```python
from build123d import *

# Parameters (mm, degrees)
SKETCH1_W            = 6.266
SKETCH1_H            = 19.6
SKETCH1_R            = 1.675
SKETCH1_W_2          = 52.832
SKETCH1_H_2          = 5
BOSS_EXTRUDE2_DEPTH  = 3.175
SKETCH3_W            = 30
SKETCH3_H            = 29.6
BOSS_EXTRUDE3_DEPTH  = 3.175
SKETCH4_R            = 4.75
CUT_EXTRUDE1_DEPTH   = 10
BOSS_EXTRUDE14_DEPTH = 3.175
CUT_EXTRUDE8_DEPTH   = 10
SKETCH24_R           = 1.475
CUT_EXTRUDE9_DEPTH   = 10
SKETCH25_R           = 3.675
SKETCH25_R_2         = 1.675
BOSS_EXTRUDE15_DEPTH = 3.175
SKETCH26_R           = 1.475
CUT_EXTRUDE12_DEPTH  = 3.175
CUT_EXTRUDE13_DEPTH  = 10
SKETCH28_R           = 3.675
SKETCH28_R_2         = 1.675
BOSS_EXTRUDE16_DEPTH = 3.175
SKETCH29_R           = 1.475
BOSS_EXTRUDE17_DEPTH = 3.175
SKETCH30_W           = 52.236337303
SKETCH30_H           = 21.491937942
BOSS_EXTRUDE18_DEPTH = 3.175
CUT_EXTRUDE14_DEPTH  = 10
SKETCH32_R           = 1.475
BOSS_EXTRUDE19_DEPTH = 4
SKETCH33_R           = 2.220955703
SKETCH33_R_2         = 1.475
SKETCH33_R_3         = 2.214708119
BOSS_EXTRUDE20_DEPTH = 3.175
SKETCH34_R           = 1.475
BOSS_EXTRUDE21_DEPTH = 4


with BuildPart() as part:
    # Sketch1 → Boss-Extrude2 (new body)
    # profile 1 of 4: a face of its own
    with BuildSketch(Plane.XY):
        with Locations((-23.283, 0)):
            Rectangle(SKETCH1_W, SKETCH1_H)
        with Locations((-23.95, -4.974)):
            Circle(SKETCH1_R, mode=Mode.SUBTRACT)
        with Locations((-23.95, 4.974)):
            Circle(SKETCH1_R, mode=Mode.SUBTRACT)
    # profile 2 of 4: a face of its own
    with BuildSketch(Plane.XY):
        with Locations((0, -12.3)):
            Rectangle(SKETCH1_W_2, SKETCH1_H_2)
    # profile 3 of 4: a face of its own
    with BuildSketch(Plane.XY):
        with Locations((0, 12.3)):
            Rectangle(SKETCH1_W_2, SKETCH1_H_2)
    # profile 4 of 4: a face of its own
    with BuildSketch(Plane.XY):
        with Locations((23.283, 0)):
            Rectangle(SKETCH1_W, SKETCH1_H)
        with Locations((23.95, -4.974)):
            Circle(SKETCH1_R, mode=Mode.SUBTRACT)
        with Locations((23.95, 4.974)):
            Circle(SKETCH1_R, mode=Mode.SUBTRACT)
    extrude(amount=BOSS_EXTRUDE2_DEPTH)

    # Sketch3 → Boss-Extrude3 (add)
    with BuildSketch(Plane.XY.offset(3.175)):
        with Locations((41.416, 0)):
            Rectangle(SKETCH3_W, SKETCH3_H)
    extrude(amount=-BOSS_EXTRUDE3_DEPTH)

    # Sketch4 → Cut-Extrude1 (cut)
    with BuildSketch(Plane(origin=(0, 0, 0), x_dir=(-1, 0, 0), z_dir=(0, 0, -1))):
        with Locations((-40.576, 7.77)):
            Circle(SKETCH4_R)
    extrude(amount=-CUT_EXTRUDE1_DEPTH, mode=Mode.SUBTRACT)

    # Sketch22 → Boss-Extrude14 (add)
    with BuildSketch(Plane(origin=(0, 0, 0), x_dir=(-1, 0, 0), z_dir=(0, 0, -1))):
        with BuildLine():
            ThreePointArc((-34.680262133, 14.8), (-40.576, 16.945), (-46.471737867, 14.8))
            Line((-46.471737867, 14.8), (-34.680262133, 14.8))
        make_face()
    extrude(amount=-BOSS_EXTRUDE14_DEPTH)

    # Sketch23 → Cut-Extrude8 (cut)
    with BuildSketch(Plane(origin=(0, 0, 0), x_dir=(-1, 0, 0), z_dir=(0, 0, -1))):
        with BuildLine():
            Line((-49.751, -14.8), (-49.751, 7.77))
            ThreePointArc((-49.751, 7.77), (-48.890866804, 11.648609936), (-46.471737867, 14.8))
            Line((-46.471737867, 14.8), (-56.416, 14.8))
            Line((-56.416, 14.8), (-56.416, -14.8))
            Line((-56.416, -14.8), (-49.751, -14.8))
        make_face()
    extrude(amount=-CUT_EXTRUDE8_DEPTH, mode=Mode.SUBTRACT)

    # Sketch24 → Cut-Extrude9 (cut)
    with BuildSketch(Plane(origin=(0, 0, 0), x_dir=(-1, 0, 0), z_dir=(0, 0, -1))):
        with Locations((23.736, 13.59)):
            Circle(SKETCH24_R)
    extrude(amount=-CUT_EXTRUDE9_DEPTH, mode=Mode.SUBTRACT)

    # Sketch25 → Boss-Extrude15 (add)
    # profile 1 of 3: a face of its own
    with BuildSketch(Plane(origin=(0, 0, 0), x_dir=(-1, 0, 0), z_dir=(0, 0, -1))):
        with Locations((23.95, -4.974)):
            Circle(SKETCH25_R)
        with Locations(Location((23.95, -4.974, 0), (0, 0, 180))):
            Circle(SKETCH25_R_2, mode=Mode.SUBTRACT)
    # profile 2 of 3: a face of its own
    with BuildSketch(Plane(origin=(0, 0, 0), x_dir=(-1, 0, 0), z_dir=(0, 0, -1))):
        with Locations((23.95, 4.974)):
            Circle(SKETCH25_R)
        with Locations(Location((23.95, 4.974, 0), (0, 0, 180))):
            Circle(SKETCH25_R_2, mode=Mode.SUBTRACT)
    # profile 3 of 3: a face of its own
    with BuildSketch(Plane(origin=(0, 0, 0), x_dir=(-1, 0, 0), z_dir=(0, 0, -1))):
        with Locations((23.736, 13.59)):
            Circle(SKETCH25_R)
        with Locations((23.736, 13.59)):
            Circle(SKETCH25_R_2, mode=Mode.SUBTRACT)
    extrude(amount=-BOSS_EXTRUDE15_DEPTH)

    # Sketch26 → Cut-Extrude12 (cut)
    with BuildSketch(Plane(origin=(0, 0, 0), x_dir=(-1, 0, 0), z_dir=(0, 0, -1))):
        with Locations((-46.076, -11.125)):
            Circle(SKETCH26_R)
    extrude(amount=-CUT_EXTRUDE12_DEPTH, mode=Mode.SUBTRACT)

    # Sketch27 → Cut-Extrude13 (cut)
    with BuildSketch(Plane(origin=(0, 0, 0), x_dir=(-1, 0, 0), z_dir=(0, 0, -1))):
        with BuildLine():
            ThreePointArc((-22.190754209, 13.59), (-22.358119678, 14.272434563), (-22.822234796, 14.8))
            Line((-22.822234796, 14.8), (-24.509273622, 14.8))
            ThreePointArc((-24.509273622, 14.8), (-24.348188772, 12.282365469), (-22.190754209, 13.59))
        make_face()
        with BuildLine():
            Line((-24.509273622, 14.8), (-22.822234796, 14.8))
            ThreePointArc((-22.822234796, 14.8), (-23.665754209, 15.065), (-24.509273622, 14.8))
        make_face()
    extrude(amount=-CUT_EXTRUDE13_DEPTH, mode=Mode.SUBTRACT)

    # Sketch28 → Boss-Extrude16 (add)
    with BuildSketch(Plane(origin=(0, 0, 0), x_dir=(-1, 0, 0), z_dir=(0, 0, -1))):
        with Locations((-23.665754209, 13.59)):
            Circle(SKETCH28_R)
        with Locations((-23.665754209, 13.59)):
            Circle(SKETCH28_R_2, mode=Mode.SUBTRACT)
    extrude(amount=-BOSS_EXTRUDE16_DEPTH)

    # Sketch29 → Boss-Extrude17 (add)
    with BuildSketch(Plane(origin=(0, 0, 0), x_dir=(-1, 0, 0), z_dir=(0, 0, -1))):
        with BuildLine():
            ThreePointArc((35.566, -11.125), (32.517318638, -5.113632727), (26.416, -2.249212118))
            Line((26.416, -2.249212118), (26.416, -14.8))
            Line((26.416, -14.8), (32.091, -14.6))
            ThreePointArc((32.091, -14.6), (34.548196065, -13.582196065), (35.566, -11.125))
        make_face()
        with Locations((32.091, -11.125)):
            Circle(SKETCH29_R, mode=Mode.SUBTRACT)
    extrude(amount=-BOSS_EXTRUDE17_DEPTH)

    # Sketch30 → Boss-Extrude18 (add)
    with BuildSketch(Plane(origin=(0, 0, 0), x_dir=(-1, 0, 0), z_dir=(0, 0, -1))):
        with Locations((-0.180648482, 0.066835569)):
            Rectangle(SKETCH30_W, SKETCH30_H)
    extrude(amount=-BOSS_EXTRUDE18_DEPTH)

    # Sketch31 → Cut-Extrude14 (cut)
    with BuildSketch(Plane(origin=(0, 0, 0), x_dir=(-1, 0, 0), z_dir=(0, 0, -1))):
        Polygon((26.416, 9.86570219), (26.416, 0.686094798), (31.474426215, 3.163131713), align=None)
    extrude(amount=-CUT_EXTRUDE14_DEPTH, mode=Mode.SUBTRACT)

    # Sketch32 → Boss-Extrude19 (add)
    with BuildSketch(Plane(origin=(0, -14.8, 0), x_dir=(-1, 0, 0), z_dir=(0, -1, 0))):
        with BuildLine():
            ThreePointArc((-22.83, -3.175), (-16.387108849, -7.772233652), (-8.83, -10.125))
            ThreePointArc((-8.83, -10.125), (-1.272891151, -7.772233652), (5.17, -3.175))
            Line((5.17, -3.175), (-22.83, -3.175))
        make_face()
        with Locations(Location((-8.83, -6.65, 0), (0, 0, 180))):
            Circle(SKETCH32_R, mode=Mode.SUBTRACT)
    extrude(amount=-BOSS_EXTRUDE19_DEPTH)

    # Sketch33 → Boss-Extrude20 (add)
    # profile 1 of 2: a face of its own
    with BuildSketch(Plane(origin=(0, 0, 0), x_dir=(-1, 0, 0), z_dir=(0, 0, -1))):
        with Locations((-23.665754209, 13.59)):
            Circle(SKETCH33_R)
        with Locations((-23.665754209, 13.59)):
            Circle(SKETCH33_R_2, mode=Mode.SUBTRACT)
    # profile 2 of 2: a face of its own
    with BuildSketch(Plane(origin=(0, 0, 0), x_dir=(-1, 0, 0), z_dir=(0, 0, -1))):
        with Locations((23.736, 13.59)):
            Circle(SKETCH33_R_3)
        with Locations((23.736, 13.59)):
            Circle(SKETCH33_R_2, mode=Mode.SUBTRACT)
    extrude(amount=-BOSS_EXTRUDE20_DEPTH)

    # Sketch34 → Boss-Extrude21 (add)
    with BuildSketch(Plane(origin=(0, -14.8, 0), x_dir=(-1, 0, 0), z_dir=(0, -1, 0))):
        with BuildLine():
            Line((5.17, -3.175), (-22.83, -3.175))
            ThreePointArc((-22.83, -3.175), (-8.83, -10.125), (5.17, -3.175))
        make_face()
        with Locations(Location((-8.83, -6.65, 0), (0, 0, 180))):
            Circle(SKETCH34_R, mode=Mode.SUBTRACT)
    extrude(amount=-BOSS_EXTRUDE21_DEPTH)


solid = part.part
```
For this review, take the finished solid that the model builds, in its own axes (mm). A direction names the side the tool comes from. Round coordinates to 2 decimals unless told otherwise and drop trailing zeros. Write each loop counter-clockwise with the first axis right and the second up, starting at its lowest first coordinate (ties: lowest second). Pieces come first, ordered by that corner, then holes. Notation, with made-up numbers: (56, -16.5) - (110, -16.5) arc R9 ccw to (110, -12.5) - close; hole circle Ø9 at (42.25, -17). An arc over 180 degrees is marked (long way). Answer as a JSON object with one key per item and string values.
1. We need section B-B on y = 5.5. Give the boundary of the cut face in (x, z) (3 decimals), then the cut area to 3 significant figures.
Response values:
{"outline": "(-26.416, 0) - (36.404, 0) - (36.404, 3.175) - (-26.416, 3.175) - close; (44.748, 0) - (49.751, 0) - (49.751, 3.175) - (44.748, 3.175) - close", "area": "215 mm2"}
2. Draft analysis for pull direction Z (two halves, no side actions). For faces 1 (the face through (-25.717, 16.685, 1.565)), 2 (the face through (8, 1, 3.175)), 3 (the face through (10.2, -12.8, 6.1)), state which applies: +Z half, -Z half, draft (parallel to the pull), parting line (faces both ways), or undercut.
Response values:
{"face 1": "draft", "face 2": "+Z half", "face 3": "undercut"}
3. We need section A-A on x = 8.83. Give the boundary of the cut face in (y, z) (3 decimals), then the cut area to 3 significant figures.
Response values:
{"outline": "(-14.8, 0) - (14.8, 0) - (14.8, 3.175) - (-10.8, 3.175) - (-10.8, 5.175) - (-14.8, 5.175) - close; (-14.8, 8.125) - (-10.8, 8.125) - (-10.8, 10.125) - (-14.8, 10.125) - close", "area": "110 mm2"}
4. Tool access review of faces 4 (the face through (0, 14.8, 2)), 5 (the face through (-26.416, 4, 2)), 6 (the face through (11, -14.8, 3)): name each direction out of +Z, -Z, +X, -X, +Y, -Y from which nothing blocks a thin tool from reaching the whole face with its end or side.
Response values:
{"face 4": "+Z, -Z, +Y", "face 5": "+Z, -Z, -X", "face 6": "+Z, -Z, +X, -X, -Y"}
5. To check wall thickness, follow line 1 along X through (y, z) = (14, 2.25); line 2 along X through (y, z) = (13.59, 2.2); line 3 along Z through (x, y) = (-16.5, 3) (3 decimals). State the ranges of each line that lie inside material, in increasing order.
Response values:
{"line 1": "x = -27.39 to -25.15, -22.32 to 22.25, 25.08 to 47.31", "line 2": "x = -27.41 to -25.21, -22.26 to 22.19, 25.14 to 47.67", "line 3": "z = 0 to 3.175"}
6. For pin 1 Ø8 at (x, y) = (-10, -10.5) entering from -Z; pin 2 Ø5.5 at (x, z) = (11.5, 6.5) entering from +Y; pin 3 Ø3.5 at (x, y) = (46.076, -11.125) entering from +Z (3 decimals); pin 4 Ø1 at (x, z) = (30, 1) entering from +Y, all flat-tipped, find the tip position at first contact; note any pin that passes through.
Response values:
{"pin 1": "stops at z = 0", "pin 2": "stops at y = -10.8", "pin 3": "stops at z = 3.175", "pin 4": "stops at y = 14.8"}
7. We need section C-C on z = 6.65. Give the boundary of the cut face in (x, y) (3 decimals), then the cut area to 3 significant figures.
Response values:
{"outline": "(-1.662, -14.8) - (7.355, -14.8) - (7.355, -10.8) - (-1.662, -10.8) - close; (10.305, -14.8) - (19.322, -14.8) - (19.322, -10.8) - (10.305, -10.8) - close", "area": "72.1 mm2"}
8. We need section D-D on z = 1.75. Give the boundary of the cut face in (x, y) (3 decimals).
Response values:
{"outline": "(-35.566, -11.125) arc R3.475 ccw to (-32.091, -14.6) - (-26.416, -14.8) - (49.751, -14.8) - (49.751, 7.77) arc R9.175 ccw to (34.68, 14.8) - (27.136, 14.8) arc R3.675 ccw to (20.196, 14.8) - (-20.266, 14.8) arc R3.675 ccw (long way) to (-26.416, 11.075) - (-26.416, -2.249) arc R10.362 ccw to start; hole circle Ø2.95 at (-32.091, -11.125); hole circle Ø2.95 at (-23.736, 13.59); hole circle Ø2.95 at (23.666, 13.59); hole circle Ø9.5 at (40.576, 7.77); hole circle Ø2.95 at (46.076, -11.125)"}
